Here's how the part is built. I have some questions about the finished solid (model axes, mm). A direction names the side the tool comes from. Round coordinates to 2 decimals unless told otherwise and drop trailing zeros. Write each loop counter-clockwise with the first axis right and the second up, starting at its lowest first coordinate (ties: lowest second). Pieces come first, ordered by that corner, then holes. Notation, with made-up numbers: (55.5, -28) - (91.5, -28) arc R21 cw to (91.5, -3) - close; hole circle Ø1 at (-39, 24.25). An arc over 180 degrees is marked (long way). One line per question, with ' | ' between items. Start each with the question number.
(1) If I drill on L1, parallel to Y at x = 0, z = -0.75; L2, parallel to X at y = -6.5, z = 4.5; L3, parallel to Z at x = 25, y = 28, over which ranges is the centre line in solid material (lowest first)?
(2) Imagine slicing it at C-C (x = -30.5). Write out the boundary of the cut face in (y, z), plus the area to 3 significant figures.
(3) Imagine slicing it at D-D (y = -37). Write out the boundary of the cut face in (x, z), plus the area to 3 significant figures.
(4) For faces 4 (the flat face through (-7.22, 26.94, -0.06)), 5 (the flat face through (-7.276, -27.154, 0.056)), 6 (the flat face through (-31.055, -44.602, -0.042)), 7 (the flat face through (24, 42, -3)), which set-ups out of +Z, -Z, +X, -X, +Y, -Y let a thin tool reach every point of the face, with its end or its side?
(5) Will these pins go through, and if not, where does the flat tip stop? pin 1 (16 mm diameter, centred on x = -13, y = 27, fed in from +Z); pin 2 (20.5 mm diameter, centred on x = -55.5, y = -4.5, fed in from -Z); pin 3 (9.5 mm diameter, centred on x = 47, y = 0, fed in from +Z).
(6) Imagine slicing it at A-A (x = 0). Write out the boundary of the cut face in (y, z), plus the area to 3 significant figures.
(7) Thinking about a two-plate mould opening in Y: for faces 1 (the flat face through (23.099, -49.196, -0.042)), 2 (the flat face through (-27.154, -7.276, -0.056)), 3 (the flat face through (15, 25, 4)), which applies, pulls with the +Y half, pulls with the -Y half, needs draft (parallel to the pull), parting line crosses it, or undercut?
from build123d import *

# Parameters (mm, degrees)
SKETCH1_R           = 20
SKETCH1_R_2         = 14
BOSS_EXTRUDE1_DEPTH = 5
BOSS_EXTRUDE2_DEPTH = 4
BOSS_EXTRUDE3_DEPTH = 3
FILLET1_R           = 0.25
FILLET6_R           = 1


with BuildPart() as part:
    # Sketch1 → Boss-Extrude1 (new, symmetric)
    with BuildSketch(Plane.XY):
        Circle(SKETCH1_R)
        Circle(SKETCH1_R_2, mode=Mode.SUBTRACT)
    extrude(amount=BOSS_EXTRUDE1_DEPTH, both=True)

    # Sketch1<3> → Boss-Extrude2 (add, symmetric)
    with BuildSketch(Plane.XY):
        with BuildLine():
            ThreePointArc((-19.318516526, -5.176380902), (-20, 0), (-19.318516526, 5.176380902))
            Line((-19.318516526, 5.176380902), (-34.773329746, 9.317485624))
            ThreePointArc((-34.773329746, 9.317485624), (-36, 0), (-34.773329746, -9.317485624))
            Line((-34.773329746, -9.317485624), (-19.318516526, -5.176380902))
        make_face()
        with BuildLine():
            ThreePointArc((-14.142135624, 14.142135624), (-10, 17.320508076), (-5.176380902, 19.318516526))
            Line((-5.176380902, 19.318516526), (-9.317485624, 34.773329746))
            ThreePointArc((-9.317485624, 34.773329746), (-18, 31.176914536), (-25.455844123, 25.455844123))
            Line((-25.455844123, 25.455844123), (-14.142135624, 14.142135624))
        make_face()
        with BuildLine():
            ThreePointArc((5.176380902, 19.318516526), (10, 17.320508076), (14.142135624, 14.142135624))
            Line((14.142135624, 14.142135624), (25.455844123, 25.455844123))
            ThreePointArc((25.455844123, 25.455844123), (18, 31.176914536), (9.317485624, 34.773329746))
            Line((9.317485624, 34.773329746), (5.176380902, 19.318516526))
        make_face()
        with BuildLine():
            Line((34.773329746, 9.317485624), (19.318516526, 5.176380902))
            ThreePointArc((19.318516526, 5.176380902), (19.828897227, 2.610523844), (20, 0))
            ThreePointArc((20, 0), (19.828897227, -2.610523844), (19.318516526, -5.176380902))
            Line((19.318516526, -5.176380902), (34.773329746, -9.317485624))
            ThreePointArc((34.773329746, -9.317485624), (36, 0), (34.773329746, 9.317485624))
        make_face()
        with BuildLine():
            Line((25.455844123, -25.455844123), (14.142135624, -14.142135624))
            ThreePointArc((14.142135624, -14.142135624), (10, -17.320508076), (5.176380902, -19.318516526))
            Line((5.176380902, -19.318516526), (9.317485624, -34.773329746))
            ThreePointArc((9.317485624, -34.773329746), (18, -31.176914536), (25.455844123, -25.455844123))
        make_face()
        with BuildLine():
            Line((-9.317485624, -34.773329746), (-5.176380902, -19.318516526))
            ThreePointArc((-5.176380902, -19.318516526), (-10, -17.320508076), (-14.142135624, -14.142135624))
            Line((-14.142135624, -14.142135624), (-25.455844123, -25.455844123))
            ThreePointArc((-25.455844123, -25.455844123), (-18, -31.176914536), (-9.317485624, -34.773329746))
        make_face()
    extrude(amount=BOSS_EXTRUDE2_DEPTH, both=True)

    # Sketch1<4> → Boss-Extrude3 (add, symmetric)
    with BuildSketch(Plane.XY):
        with BuildLine():
            ThreePointArc((-9.317485624, 34.773329746), (-18, 31.176914536), (-25.455844123, 25.455844123))
            Line((-25.455844123, 25.455844123), (-36.5, 63.219854476))
            Line((-36.5, 63.219854476), (-9.317485624, 34.773329746))
        make_face()
        with BuildLine():
            ThreePointArc((25.455844123, 25.455844123), (18, 31.176914536), (9.317485624, 34.773329746))
            Line((9.317485624, 34.773329746), (36.5, 63.219854476))
            Line((36.5, 63.219854476), (25.455844123, 25.455844123))
        make_face()
        with BuildLine():
            ThreePointArc((34.773329746, -9.317485624), (36, 0), (34.773329746, 9.317485624))
            Line((34.773329746, 9.317485624), (73, 0))
            Line((73, 0), (34.773329746, -9.317485624))
        make_face()
        with BuildLine():
            ThreePointArc((9.317485624, -34.773329746), (18, -31.176914536), (25.455844123, -25.455844123))
            Line((25.455844123, -25.455844123), (36.5, -63.219854476))
            Line((36.5, -63.219854476), (9.317485624, -34.773329746))
        make_face()
        with BuildLine():
            ThreePointArc((-25.455844123, -25.455844123), (-18, -31.176914536), (-9.317485624, -34.773329746))
            Line((-9.317485624, -34.773329746), (-36.5, -63.219854476))
            Line((-36.5, -63.219854476), (-25.455844123, -25.455844123))
        make_face()
        with BuildLine():
            ThreePointArc((-34.773329746, 9.317485624), (-36, 0), (-34.773329746, -9.317485624))
            Line((-34.773329746, -9.317485624), (-73, 0))
            Line((-73, 0), (-34.773329746, 9.317485624))
        make_face()
    extrude(amount=BOSS_EXTRUDE3_DEPTH, both=True)

    # Fillet1
    fillet1_edges = [part.edges().sort_by_distance(p)[0] for p in [
        (-20, 0, 5),
        (-20, 0, -5),
    ]]
    fillet(fillet1_edges, radius=FILLET1_R)

    # Fillet6
    # the kernel refuses this fillet: 1 mm, written as the material it adds along each edge
    with BuildSketch(Plane(origin=(0, 0, -3), x_dir=(0.7071067811865468, 0.7071067811865483, 0), z_dir=(0.7071067811865483, -0.7071067811865468, 0))) as fillet6_piece_1_section:
        with BuildLine():
            CenterArc((36 + FILLET6_R, -FILLET6_R), FILLET6_R, 90, 90)
            Line((36 + FILLET6_R, 0), (36, 0))
            Line((36, 0), (36, -FILLET6_R))
        make_face()
    fillet6_piece_1 = revolve(axis=Axis((0, 0, -3), (0, 0, 1)), revolution_arc=30, mode=Mode.PRIVATE)
    fillet6_piece_1 = split(fillet6_piece_1, bisect_by=Plane(origin=(11.853809218, 37.427594574, -3.280987198), z_dir=(0.722987141265996, -0.6908614865253547, 0)), keep=Keep.TOP, mode=Mode.PRIVATE)
    fillet6_piece_1 = split(fillet6_piece_1, bisect_by=Plane(origin=(26.486343095, 28.979497201, -3.280987198), z_dir=(-0.9597971684602362, 0.28069448768316235, 0)), keep=Keep.TOP, mode=Mode.PRIVATE)
    add(fillet6_piece_1)
    # the kernel refuses this fillet: 1 mm, written as the material it takes off along each edge
    with BuildSketch(Plane(origin=(0, 0, -4), x_dir=(0.9456375488425219, -0.325222425762903, 0), z_dir=(-0.325222425762903, -0.9456375488425219, 0))) as fillet6_2_piece_1:
        with BuildLine():
            CenterArc((36 - FILLET6_R, FILLET6_R), FILLET6_R, 270, 90)
            Line((36 - FILLET6_R, 0), (36, 0))
            Line((36, 0), (36, FILLET6_R))
        make_face()
    revolve(axis=Axis((0, 0, -4), (0, 0, 1)), revolution_arc=37.958102254, mode=Mode.SUBTRACT)
    with BuildSketch(Plane(origin=(0, 0, -4), x_dir=(0.19116789183018731, -0.9815573529515235, 0), z_dir=(-0.9815573529515235, -0.19116789183018731, 0))) as fillet6_2_piece_2:
        with BuildLine():
            CenterArc((36 - FILLET6_R, FILLET6_R), FILLET6_R, 270, 90)
            Line((36, FILLET6_R), (36, 0))
            Line((36, 0), (36 - FILLET6_R, 0))
        make_face()
    revolve(axis=Axis((0, 0, -4), (0, 0, 1)), revolution_arc=37.958102254, mode=Mode.SUBTRACT)
    with BuildSketch(Plane(origin=(0, 0, -4), x_dir=(-0.7544696570123329, -0.6563349271886211, 0), z_dir=(-0.6563349271886211, 0.7544696570123329, 0))) as fillet6_2_piece_3:
        with BuildLine():
            CenterArc((36 - FILLET6_R, FILLET6_R), FILLET6_R, 270, 90)
            Line((36, FILLET6_R), (36, 0))
            Line((36, 0), (36 - FILLET6_R, 0))
        make_face()
    revolve(axis=Axis((0, 0, -4), (0, 0, 1)), revolution_arc=37.958102254, mode=Mode.SUBTRACT)
    with BuildSketch(Plane(origin=(0, 0, -4), x_dir=(-0.9456375488425217, 0.32522242576290356, 0), z_dir=(0.32522242576290356, 0.9456375488425217, 0))) as fillet6_2_piece_4:
        with BuildLine():
            CenterArc((36 - FILLET6_R, FILLET6_R), FILLET6_R, 270, 90)
            Line((36 - FILLET6_R, 0), (36, 0))
            Line((36, 0), (36, FILLET6_R))
        make_face()
    revolve(axis=Axis((0, 0, -4), (0, 0, 1)), revolution_arc=37.958102254, mode=Mode.SUBTRACT)
    with BuildSketch(Plane(origin=(0, 0, -4), x_dir=(-0.19116789183018898, 0.9815573529515234, 0), z_dir=(0.9815573529515234, 0.19116789183018898, 0))) as fillet6_2_piece_5:
        with BuildLine():
            CenterArc((36 - FILLET6_R, FILLET6_R), FILLET6_R, 270, 90)
            Line((36 - FILLET6_R, 0), (36, 0))
            Line((36, 0), (36, FILLET6_R))
        make_face()
    revolve(axis=Axis((0, 0, -4), (0, 0, 1)), revolution_arc=37.958102254, mode=Mode.SUBTRACT)


solid = part.part
Check sheet entries:
1) L1: -20 to -14, 14 to 20 | L2: -18.91 to -12.4, 12.4 to 18.91 | L3: -3 to 3
2) outline: (-56.94, -3) - (-42.7, -3) - (-42.7, 3) - (-56.94, 3) - close; (-8.17, -4) - (8.17, -4) - (8.17, 4) - (-8.17, 4) - close; (42.7, -3) - (56.94, -3) - (56.94, 3) - (42.7, 3) - close | area: 302 mm^2
3) outline: (-28.83, -3) - (-11.45, -3) - (-11.45, 3) - (-28.83, 3) - close; (11.45, -3) - (28.83, -3) - (28.83, 3) - (11.45, 3) - close | area: 209 mm^2
4) face 4: +Z, -Z, +Y | face 5: +Z, -Z, -Y | face 6: +Z, -Z, -X | face 7: -Z, +X, +Y
5) pin 1: z = 4 | pin 2: z = -3 | pin 3: z = 3
6) outline: (-20, -4.75) arc R0.25 ccw to (-19.75, -5) - (-14, -5) - (-14, 5) - (-19.75, 5) arc R0.25 ccw to (-20, 4.75) - close; (14, -5) - (19.75, -5) arc R0.25 ccw to (20, -4.75) - (20, 4.75) arc R0.25 ccw to (19.75, 5) - (14, 5) - close | area: 120 mm^2
7) face 1: pulls with the -Y half | face 2: undercut | face 3: needs draft
